from build123d import *

# Parameters (mm, degrees)
SKETCH1_W                = 26
SKETCH1_H                = 25.3
BOSS_EXTRUDE1_DEPTH      = 1.5
SKETCH2_W                = 14.8
SKETCH2_H                = 3
CUT_EXTRUDE1_DEPTH       = 1.5
SKETCH3_R                = 1.15
CUT_EXTRUDE2_DEPTH       = 1.5
SKETCH4_R                = 1.75
SKETCH4_R_2              = 1.15
BOSS_EXTRUDE3_DEPTH      = 0.1
BOSS_EXTRUDE3_DEPTH_BACK = 1.6
SKETCH6_W                = 24.8
SKETCH6_H                = 16.7
BOSS_EXTRUDE4_DEPTH      = 1.7
SKETCH7_W                = 21.1
SKETCH7_H                = 3.3
SKETCH7_W_2              = 12.9
BOSS_EXTRUDE5_DEPTH      = 0.8
SKETCH8_R                = 0.65
CUT_EXTRUDE4_DEPTH       = 4.2


with BuildPart() as part:
    # Sketch1 → Boss-Extrude1 (new body)
    with BuildSketch(Plane(origin=(0, 0, 0), x_dir=(1, 0, 0), z_dir=(0, 1, 0))):
        with Locations((2.394736842, -5.260526316)):
            Rectangle(SKETCH1_W, SKETCH1_H)
    extrude(amount=BOSS_EXTRUDE1_DEPTH)

    # Sketch2 → Cut-Extrude1 (cut)
    with BuildSketch(Plane(origin=(0, 1.5, 0), x_dir=(1, 0, 0), z_dir=(0, 1, 0))):
        with Locations((2.394736842, -16.410526316)):
            Rectangle(SKETCH2_W, SKETCH2_H)
    extrude(amount=-CUT_EXTRUDE1_DEPTH, mode=Mode.SUBTRACT)

    # Sketch3 → Cut-Extrude2 (cut)
    with BuildSketch(Plane(origin=(0, 1.5, 0), x_dir=(1, 0, 0), z_dir=(0, 1, 0))):
        with Locations((-8.455263158, 5.239473684)):
            Circle(SKETCH3_R)
        with Locations((13.244736842, 5.239473684)):
            Circle(SKETCH3_R)
        with Locations((13.244736842, -15.760526316)):
            Circle(SKETCH3_R)
        with Locations((-8.455263158, -15.760526316)):
            Circle(SKETCH3_R)
    extrude(amount=-CUT_EXTRUDE2_DEPTH, mode=Mode.SUBTRACT)

    # Sketch4 → Boss-Extrude3 (add, two sides)
    with BuildSketch(Plane(origin=(0, 1.5, 0), x_dir=(1, 0, 0), z_dir=(0, 1, 0))) as boss_extrude3_sk:
        with Locations((-8.455263158, 5.239473684)):
            Circle(SKETCH4_R)
        with Locations((-8.455263158, 5.239473684)):
            Circle(SKETCH4_R_2, mode=Mode.SUBTRACT)
        with Locations((13.244736842, 5.239473684)):
            Circle(SKETCH4_R)
        with Locations((13.244736842, 5.239473684)):
            Circle(SKETCH4_R_2, mode=Mode.SUBTRACT)
        with Locations((13.244736842, -15.760526316)):
            Circle(SKETCH4_R)
        with Locations((13.244736842, -15.760526316)):
            Circle(SKETCH4_R_2, mode=Mode.SUBTRACT)
        with Locations((-8.455263158, -15.760526316)):
            Circle(SKETCH4_R)
        with Locations((-8.455263158, -15.760526316)):
            Circle(SKETCH4_R_2, mode=Mode.SUBTRACT)
    extrude(amount=BOSS_EXTRUDE3_DEPTH)
    extrude(boss_extrude3_sk.sketch, amount=-BOSS_EXTRUDE3_DEPTH_BACK)

    # Sketch6 → Boss-Extrude4 (add)
    with BuildSketch(Plane(origin=(0, 1.5, 0), x_dir=(1, 0, 0), z_dir=(0, 1, 0))):
        with Locations((2.394736842, -5.160526316)):
            Rectangle(SKETCH6_W, SKETCH6_H)
    extrude(amount=BOSS_EXTRUDE4_DEPTH)

    # Sketch7 → Boss-Extrude5 (add)
    with BuildSketch(Plane.XZ):
        with Locations((2.394736842, 3.960526316)):
            Rectangle(SKETCH7_W, SKETCH7_H)
        with Locations((3.144736842, -2.039473684)):
            Rectangle(SKETCH7_W_2, SKETCH7_H)
    extrude(amount=BOSS_EXTRUDE5_DEPTH)

    # Sketch8 → Cut-Extrude4 (cut, through all)
    with BuildSketch(Plane.XZ):
        with Locations((-1.955263158, -6.241133994)):
            Circle(SKETCH8_R)
        with Locations((0.944736842, -6.241133994)):
            Circle(SKETCH8_R)
        with Locations((3.844736842, -6.241133994)):
            Circle(SKETCH8_R)
        with Locations((6.744736842, -6.241133994)):
            Circle(SKETCH8_R)
    extrude(amount=-CUT_EXTRUDE4_DEPTH, mode=Mode.SUBTRACT)


solid = part.part
Geometry check sheet. Reference: the model listing, model coordinates, mm. A direction names the side the tool comes from. Give positions to 0.01 mm unless a question says otherwise; leave off trailing zeros. Loops run counter-clockwise (first coordinate to the right, second up) from the corner with the lowest first, then second, coordinate; pieces in that order, holes last. Notation, with made-up numbers: M 41.25,73 L 83.25,73 A20 cw 83.25,112 Z; hole C 45.5,23.25 d8. An arc over 180 degrees is marked long. Write each question's results on one line, items separated by ' | '.
1) Section check B-B, the plane x = 1.25. Record the boundary of the cut face in (y, z) (3 decimals).
Answers follow:
outline: M -0.8,-3.689 L 0,-3.689 L 0,-5.667 L 1.5,-5.667 L 1.5,-3.189 L 3.2,-3.189 L 3.2,13.511 L 1.5,13.511 L 1.5,14.911 L 0,14.911 L 0,5.611 L -0.8,5.611 L -0.8,2.311 L 0,2.311 L 0,-0.389 L -0.8,-0.389 Z; M 0,-7.389 L 1.5,-7.389 L 1.5,-6.815 L 0,-6.815 Z
2) Thickness scan on line 1 (X direction, y = 1.2, z = 16.75); line 2 (Z direction, x = 1.75, y = 2.95); line 3 (Z direction, x = -4, y = 0.1). Record the ranges inside material, lowest first.
Answers follow:
line 1: -10.61 to -9.04, -7.87 to -5.01, 9.79 to 12.66, 13.83 to 15.39 | line 2: -3.19 to 13.51 | line 3: -7.39 to 14.91
3) Section check C-C, the plane z = 7.5. Record the boundary of the cut face in (x, y).
Answers follow:
outline: M -10.61,0 L 15.39,0 L 15.39,1.5 L 14.79,1.5 L 14.79,3.2 L -10.01,3.2 L -10.01,1.5 L -10.61,1.5 Z
4) Tool access check on faces 1 (the face through (-5.005, 1, 16)), 2 (the face through (-7, 1.6, 16)), 3 (the face through (14, 1.6, -4)). Record the directions out of +Z, -Z, +X, -X, +Y, -Y that give a thin tool (end or side, any length) a straight path to the whole face; none if there is none.
Answers follow:
face 1: +Z, +Y, -Y | face 2: +Z, +X, -X, +Y | face 3: -Z, +X, -X, +Y
5) Section check A-A, the plane y = -0.4. Record the boundary of the cut face in (x, z), plus the area to 3 significant figures.
Answers follow:
outline: M -8.16,2.31 L 12.94,2.31 L 12.94,5.61 L -8.16,5.61 Z; M -3.31,-3.69 L 9.59,-3.69 L 9.59,-0.39 L -3.31,-0.39 Z | area: 112 mm2
6) Gauge pin test, flat ends, axial feed: pin 1 (0.8 mm diameter, centred on x = 4.5, y = 2.5, fed in from +Z); pin 2 (1.5 mm diameter, centred on x = -3.5, z = -4, fed in from +Y); pin 3 (0.9 mm diameter, centred on x = -1, y = -0.5, fed in from -Z); pin 4 (1.4 mm diameter, centred on x = 13.24, z = 15.76, fed in from +Y). Record the tip position at first contact, or that the pin passes through.
Answers follow:
pin 1: z = 13.51 | pin 2: y = 1.5 | pin 3: z = -3.69 | pin 4: through
7) Section check D-D, the plane x = 5. Record the boundary of the cut face in (y, z).
Answers follow:
outline: M -0.8,-3.69 L 0,-3.69 L 0,-7.39 L 1.5,-7.39 L 1.5,-3.19 L 3.2,-3.19 L 3.2,13.51 L 1.5,13.51 L 1.5,14.91 L 0,14.91 L 0,5.61 L -0.8,5.61 L -0.8,2.31 L 0,2.31 L 0,-0.39 L -0.8,-0.39 Z
